```python
from build123d import *

# Parameters (mm, degrees)
BOSS_EXTRUDE1_DEPTH         = 22.5
M5_TAPPED_HOLE1_D           = 4.2
M5_TAPPED_HOLE1_DEPTH       = 12.4
M5_TAPPED_HOLE1_CSINK_D     = 5.05
M5_TAPPED_HOLE1_CSINK_ANGLE = 90
M5_TAPPED_HOLE1_TIP         = 1.2618073
M4X0_7_TAPPED_HOLE1_D       = 3.3
M4X0_7_TAPPED_HOLE1_DEPTH   = 10.1
M4X0_7_TAPPED_HOLE1_TIP     = 0.991420021
M6X1_0_TAPPED_HOLE1_D       = 5
M6X1_0_TAPPED_HOLE1_DEPTH   = 15
M6X1_0_TAPPED_HOLE1_TIP     = 1.502151548


with BuildPart() as part:
    # Sketch2 → Boss-Extrude1 (new body, symmetric)
    with BuildSketch(Plane.XY):
        with BuildLine():
            Line((13, 19), (-13, 19))
            Line((-13, 19), (-13, 20))
            Line((-13, 20), (-20.5, 20))
            Line((-20.5, 20), (-22.5, 18))
            Line((-22.5, 18), (-22.5, 10.5))
            Line((-22.5, 10.5), (-21.5, 10.5))
            Line((-21.5, 10.5), (-21.5, -13))
            Line((-21.5, -13), (-10, -13))
            Line((-10, -13), (-4.877686087, -6.340991913))
            ThreePointArc((-4.877686087, -6.340991913), (0, 8), (4.877686087, -6.340991913))
            Line((4.877686087, -6.340991913), (10, -13))
            Line((10, -13), (21.5, -13))
            Line((21.5, -13), (21.5, 10.5))
            Line((21.5, 10.5), (22.5, 10.5))
            Line((22.5, 10.5), (22.5, 18))
            Line((22.5, 18), (20.5, 20))
            Line((20.5, 20), (13, 20))
            Line((13, 20), (13, 19))
        make_face()
    extrude(amount=BOSS_EXTRUDE1_DEPTH, both=True)

    # M5 Tapped Hole1
    with Locations(Plane(origin=(0, 20, 0), x_dir=(1, 0, 0), z_dir=(0, 1, 0))):
        with Locations((-16, 15), (16, 15), (-16, -15), (16, -15)):
            CounterSinkHole(M5_TAPPED_HOLE1_D / 2, M5_TAPPED_HOLE1_CSINK_D / 2, depth=M5_TAPPED_HOLE1_DEPTH, counter_sink_angle=M5_TAPPED_HOLE1_CSINK_ANGLE)
            with Locations((0, 0, -(M5_TAPPED_HOLE1_DEPTH + M5_TAPPED_HOLE1_TIP / 2))):  # 118° drill point
                Cone(0, M5_TAPPED_HOLE1_D / 2, M5_TAPPED_HOLE1_TIP, mode=Mode.SUBTRACT)

    # M4x0.7 Tapped Hole1
    with Locations(Plane(origin=(0, 19, 0), x_dir=(1, 0, 0), z_dir=(0, 1, 0))):
        with Locations((0, 0)):
            Hole(M4X0_7_TAPPED_HOLE1_D / 2, depth=M4X0_7_TAPPED_HOLE1_DEPTH)
            with Locations((0, 0, -(M4X0_7_TAPPED_HOLE1_DEPTH + M4X0_7_TAPPED_HOLE1_TIP / 2))):  # 118° drill point
                Cone(0, M4X0_7_TAPPED_HOLE1_D / 2, M4X0_7_TAPPED_HOLE1_TIP, mode=Mode.SUBTRACT)

    # M6x1.0 Tapped Hole1
    with Locations(Plane.ZY.offset(21.5)):
        with Locations((0, 0)):
            Hole(M6X1_0_TAPPED_HOLE1_D / 2, depth=M6X1_0_TAPPED_HOLE1_DEPTH)
            with Locations((0, 0, -(M6X1_0_TAPPED_HOLE1_DEPTH + M6X1_0_TAPPED_HOLE1_TIP / 2))):  # 118° drill point
                Cone(0, M6X1_0_TAPPED_HOLE1_D / 2, M6X1_0_TAPPED_HOLE1_TIP, mode=Mode.SUBTRACT)


solid = part.part
```
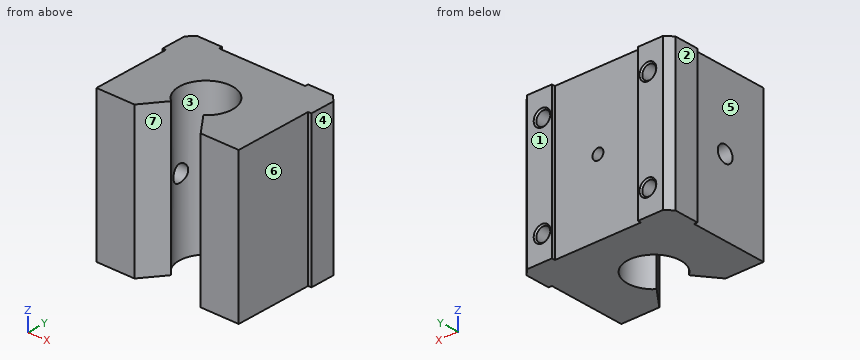
Design review of the part built by this model. Coordinates are the model's own, in mm. Face numbers are marked on the shaded views. A direction names the side the tool comes from. Round coordinates to 2 decimals unless told otherwise and drop trailing zeros. Write each loop counter-clockwise with the first axis right and the second up, starting at its lowest first coordinate (ties: lowest second). Pieces come first, ordered by that corner, then holes. Notation, with made-up numbers: (-14.5, 4.25) -> (39.5, 4.25) arc R13 cw to (39.5, 26.25) -> close; hole circle Ø9 at (-25, 48.25). An arc over 180 degrees is marked (long way). Write item = value, one per line. Start each with the question number.
1) Take a section at B-B, the plane y = 15.5. State the section outline as (x, z) points, plus the area to 3 significant figures.
2) Wall thickness on probe 1 along X at (y, z) = (13.25, -15); probe 2 along Z at (x, y) = (-16, 16.5); probe 3 along Y at (x, z) = (-12, 0): over which ranges is each line inside the solid? List them lowest first. Write a range as from..to.
3) Take a section at D-D, the plane y = -3.5. State the section outline as (x, z) points, plus the area to 3 significant figures.
4) Tool access review of the marked faces 5, 6 and 7: name each direction out of +Z, -Z, +X, -X, +Y, -Y from which nothing blocks a thin tool from reaching the whole face with its end or side.
5) Take a section at C-C, the plane z = 4. State the section outline as (x, y) points.
6) Mouldability with a two-part tool opening along X and no side actions: class the marked faces 1, 2, 3 and 4 as +X half, -X half, draft (parallel to the pull), parting line (faces both ways), or undercut.
7) Clearance check with flat-ended pins moving along their axes: pin 1 (6.5 mm diameter, centred on y = 0, z = 0, fed in from +X); pin 2 (13 mm diameter, centred on x = 0, z = 3.5, fed in from +Y); pin 3 (1.5 mm diameter, centred on y = -5.5, z = -3, fed in from -X); pin 4 (14.5 mm diameter, centred on x = 0, y = 0, fed in from +Z). State where each tip first meets the part, or that it passes through.
8) Take a section at A-A, the plane y = 0. State the section outline as (x, z) points, plus the area to 3 significant figures.
Results list:
q1.outline = (-22.5, -22.5) -> (22.5, -22.5) -> (22.5, 22.5) -> (-22.5, 22.5) -> close; hole circle Ø4.2 at (-16, -15); hole circle Ø4.2 at (-16, 15); hole circle Ø3.3 at (0, 0); hole circle Ø4.2 at (16, -15); hole circle Ø4.2 at (16, 15)
q1.area = 1,960 mm²
q2.probe_1 = -22.5..-18.1, -13.9..13.9, 18.1..22.5
q2.probe_2 = -22.5..-17.1, -12.9..12.9, 17.1..22.5
q2.probe_3 = -13..-2.5, 2.5..19
q3.outline = (-21.5, -22.5) -> (-7.19, -22.5) -> (-7.19, 22.5) -> (-21.5, 22.5) -> close; (7.19, -22.5) -> (21.5, -22.5) -> (21.5, 22.5) -> (7.19, 22.5) -> close
q3.area = 1,290 mm²
q4.face_5 = +Z, -Z, -X, -Y
q4.face_6 = +Z, -Z, +X, -Y
q4.face_7 = +Z, -Z, -Y
q5.outline = (-22.5, 10.5) -> (-21.5, 10.5) -> (-21.5, -13) -> (-10, -13) -> (-4.88, -6.34) arc R8 cw (long way) to (4.88, -6.34) -> (10, -13) -> (21.5, -13) -> (21.5, 10.5) -> (22.5, 10.5) -> (22.5, 18) -> (20.5, 20) -> (13, 20) -> (13, 19) -> (-13, 19) -> (-13, 20) -> (-20.5, 20) -> (-22.5, 18) -> close
q6.face_1 = draft
q6.face_2 = -X half
q6.face_3 = undercut
q6.face_4 = +X half
q7.pin_1 = 21.5
q7.pin_2 = 19
q7.pin_3 = -21.5
q7.pin_4 = through
q8.outline = (-21.5, -22.5) -> (-8, -22.5) -> (-8, -2.5) -> (-21.5, -2.5) -> close; (-21.5, 2.5) -> (-8, 2.5) -> (-8, 22.5) -> (-21.5, 22.5) -> close; (8, -22.5) -> (21.5, -22.5) -> (21.5, 22.5) -> (8, 22.5) -> close
q8.area = 1,150 mm²
